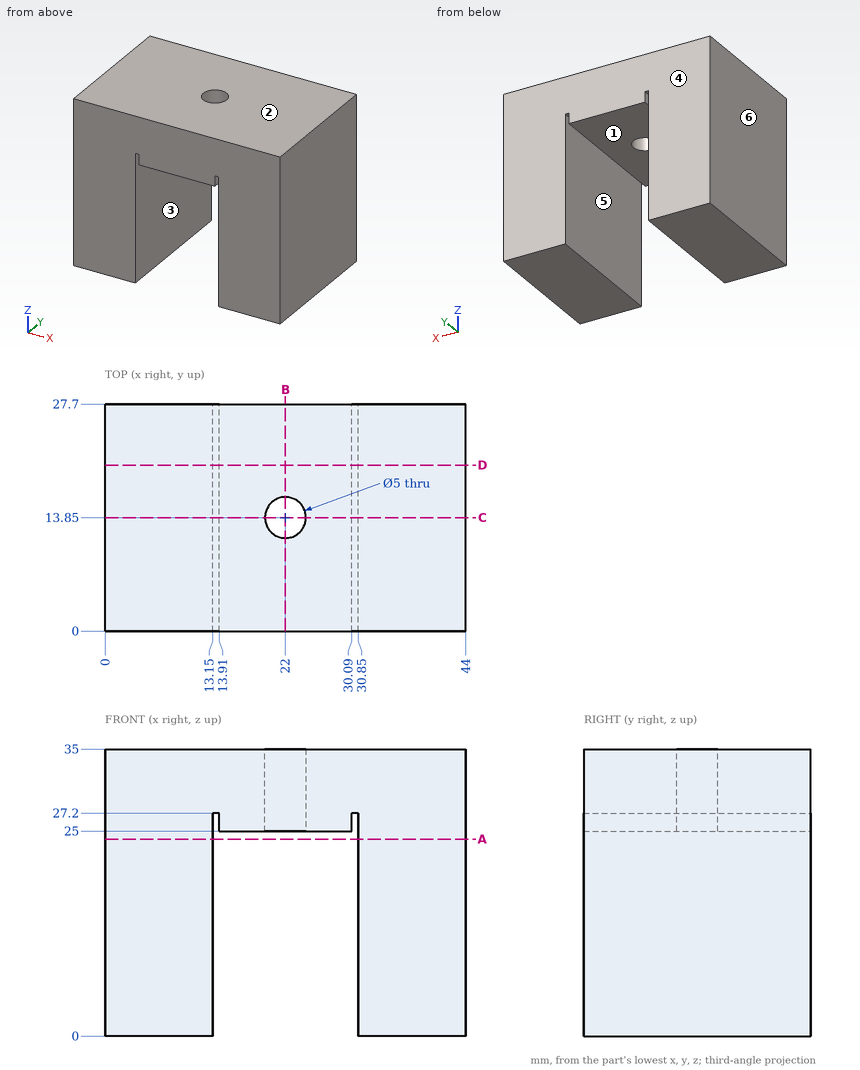
Print and shaded views of the part. All mm, measured from the part's lowest x, y and z. A direction names the side the tool comes from. Round coordinates to 2 decimals unless told otherwise and drop trailing zeros. Order: outer loops, then holes, each group sorted by start corner. A loop starts at its lowest first (then second) coordinate and runs counter-clockwise, first axis right, second up.
Q1. Slice it at A-A (z = 24). Write the cut outline in (x, y), and give its area (3 significant figures).
Q2. Slice it at D-D (y = 20.25). Write the cut outline in (x, z), and give its area (3 significant figures).
Q3. Which spindle directions (+Z, -Z, +X, -X, +Y, -Y) get a long thin tool onto all of the face, cutting with end or side? Do the marked faces 1 and 2. Say none if no direction does.
Q4. Slice it at B-B (x = 22). Write the cut outline in (y, z).
Q5. Slice it at C-C (y = 13.85). Write the cut outline in (x, z), and give its area (3 significant figures).
Q6. Drop flat-ended pins along their axis: pin 1 (8 mm diameter, centred on x = 22, y = 13.85, fed in from +Z); pin 2 (0.6 mm diameter, centred on x = 13.5, y = 14.5, fed in from -Z); pin 3 (8 mm diameter, centred on x = 23, y = 16.5, fed in from -Z). Give the stop position or say it passes through.
Q7. Two-plate mould, pull along X, no slides. Class the marked faces 3, 4, 5 and 6: pulls with the +X half, pulls with the -X half, needs draft (parallel to the pull), parting line crosses it, or undercut.
Q8. Wall check: L1, parallel to Y at x = 22, z = 29; L2, parallel to X at y = 26.5, z = 9; L3, parallel to Z at x = 26.5, y = 10.25. Give the ranges that are in metal, low to high.
Results below:
1. outline: (0, 0) - (13.15, 0) - (13.15, 27.7) - (0, 27.7) - close; (30.85, 0) - (44, 0) - (44, 27.7) - (30.85, 27.7) - close
1. area: 729 mm2
2. outline: (0, 0) - (13.15, 0) - (13.15, 27.2) - (13.91, 27.2) - (13.91, 25) - (30.09, 25) - (30.09, 27.2) - (30.85, 27.2) - (30.85, 0) - (44, 0) - (44, 35) - (0, 35) - close
2. area: 1,090 mm2
3. face 1: -Z, +Y, -Y
3. face 2: +Z, +X, -X, +Y, -Y
4. outline: (0, 25) - (11.35, 25) - (11.35, 35) - (0, 35) - close; (16.35, 25) - (27.7, 25) - (27.7, 35) - (16.35, 35) - close
5. outline: (0, 0) - (13.15, 0) - (13.15, 27.2) - (13.91, 27.2) - (13.91, 25) - (19.5, 25) - (19.5, 35) - (0, 35) - close; (24.5, 25) - (30.09, 25) - (30.09, 27.2) - (30.85, 27.2) - (30.85, 0) - (44, 0) - (44, 35) - (24.5, 35) - close
5. area: 1,040 mm2
6. pin 1: stops at z = 35
6. pin 2: stops at z = 27.2
6. pin 3: stops at z = 25
7. face 3: undercut
7. face 4: needs draft
7. face 5: undercut
7. face 6: pulls with the -X half
8. L1: y = 0 to 11.35, 16.35 to 27.7
8. L2: x = 0 to 13.15, 30.85 to 44
8. L3: z = 25 to 35
